Geometry: final body of the model. Coordinates: model frame, mm. A direction names the side the tool comes from. Coordinates: 2 decimals unless noted, no trailing zeros. Order: outer loops, then holes, each group sorted by start corner. A loop starts at its lowest first (then second) coordinate and runs counter-clockwise, first axis right, second up. Notation, with made-up numbers: M 14,28 L 19,28 A22 ccw 19,60 Z; hole C 13,25.5 d10. An arc over 180 degrees is marked long. Write item = value, one per line.
from build123d import *

# Parameters (mm, degrees)
ESQUISSE1_W             = 360
ESQUISSE1_H             = 356
BOSS_EXTRU_1_DEPTH      = 47.5
CONG_1_R                = 25
ENL_V_MAT_EXTRU_1_DEPTH = 44.5
ESQUISSE3_W             = 320
ESQUISSE3_H             = 35
ENL_V_MAT_EXTRU_2_DEPTH = 10
ESQUISSE5_W             = 40
ESQUISSE5_H             = 40
ESQUISSE5_W_2           = 34
ESQUISSE5_H_2           = 34
EXTRU_MINCE1_DEPTH      = 9.5
ESQUISSE10_W            = 34
ESQUISSE10_H            = 9.5
ENL_V_MAT_EXTRU_4_DEPTH = 10
ESQUISSE13_W            = 34
ESQUISSE13_H            = 9.5
ENL_V_MAT_EXTRU_5_DEPTH = 10


with BuildPart() as part:
    # Esquisse1 → Boss.-Extru.1 (new body)
    with BuildSketch(Plane.XY):
        with Locations((180, 178)):
            Rectangle(ESQUISSE1_W, ESQUISSE1_H)
    extrude(amount=BOSS_EXTRU_1_DEPTH)

    # Congé1
    cong_1_edges = [part.edges().sort_by_distance(p)[0] for p in [
        (0, 356, 23.75),
        (360, 356, 23.75),
        (360, 0, 23.75),
        (0, 0, 23.75),
    ]]
    fillet(cong_1_edges, radius=CONG_1_R)

    # Esquisse2 → Enlèv. mat.-Extru.1 (cut)
    with BuildSketch(Plane.XY.offset(47.5)):
        with BuildLine():
            Line((3, 331), (3, 25))
            ThreePointArc((3, 25), (9.443650814, 9.443650814), (25, 3))
            Line((25, 3), (335, 3))
            ThreePointArc((335, 3), (350.556349186, 9.443650814), (357, 25))
            Line((357, 25), (357, 331))
            ThreePointArc((357, 331), (350.556349186, 346.556349186), (335, 353))
            Line((335, 353), (25, 353))
            ThreePointArc((25, 353), (9.443650814, 346.556349186), (3, 331))
        make_face()
    extrude(amount=-ENL_V_MAT_EXTRU_1_DEPTH, mode=Mode.SUBTRACT)

    # Esquisse3 → Enlèv. mat.-Extru.2 (cut)
    with BuildSketch(Plane(origin=(0, 356, 0), x_dir=(1, 0, 0), z_dir=(0, 1, 0))):
        with Locations((180, -30)):
            Rectangle(ESQUISSE3_W, ESQUISSE3_H)
    extrude(amount=-ENL_V_MAT_EXTRU_2_DEPTH, mode=Mode.SUBTRACT)

    # Esquisse5 → Extru.-Mince1 (add)
    with BuildSketch(Plane.XY.offset(3)):
        with Locations((63, 333)):
            Rectangle(ESQUISSE5_W, ESQUISSE5_H)
        with Locations((63, 333)):
            Rectangle(ESQUISSE5_W_2, ESQUISSE5_H_2, mode=Mode.SUBTRACT)
        with Locations((297, 333)):
            Rectangle(ESQUISSE5_W, ESQUISSE5_H)
        with Locations((297, 333)):
            Rectangle(ESQUISSE5_W_2, ESQUISSE5_H_2, mode=Mode.SUBTRACT)
    extrude(amount=EXTRU_MINCE1_DEPTH)

    # Esquisse10 → Enlèv. mat.-Extru.4 (cut)
    with BuildSketch(Plane(origin=(0, 356, 0), x_dir=(1, 0, 0), z_dir=(0, 1, 0))):
        with Locations((297, -7.75)):
            Rectangle(ESQUISSE10_W, ESQUISSE10_H)
    extrude(amount=-ENL_V_MAT_EXTRU_4_DEPTH, mode=Mode.SUBTRACT)

    # Esquisse13 → Enlèv. mat.-Extru.5 (cut)
    with BuildSketch(Plane(origin=(0, 356, 0), x_dir=(1, 0, 0), z_dir=(0, 1, 0))):
        with Locations((63, -7.75)):
            Rectangle(ESQUISSE13_W, ESQUISSE13_H)
    extrude(amount=-ENL_V_MAT_EXTRU_5_DEPTH, mode=Mode.SUBTRACT)


solid = part.part
1) Section A-A, the plane y = 54. Return loops of the section in (x, z), and give its area (3 significant figures).
Numbers:
outline = M 0,0 L 360,0 L 360,47.5 L 357,47.5 L 357,3 L 3,3 L 3,47.5 L 0,47.5 Z
area = 1,350 mm²
2) Set-up query: faces 4 (the face through (352.482, 7.129, 24.082)), 5 (the face through (3, 180, 26)), 6 (the face through (63, 316, 8)). Return all of +Z, -Z, +X, -X, +Y, -Y with unobstructed straight access to the full face (end or side cutting, diameter ignored); none if empty.
Numbers:
face_4 = +Z, -Z, +X, -Y
face_5 = +Z
face_6 = +Z, +Y
3) Mould query, pull axis X, two halves, no side actions, for faces 1 (the face through (0, 176, 23)), 2 (the face through (178, 0, 23)), 3 (the face through (357, 176, 26)). Classes: pulls with the +X half, pulls with the -X half, needs draft (parallel to the pull), parting line crosses it, or undercut.
Numbers:
face_1 = pulls with the -X half
face_2 = needs draft
face_3 = undercut
4) Line query: L1, parallel to X at y = 132, z = 33; L2, parallel to Y at x = 65, z = 9.5; L3, parallel to Y at x = 186, z = 7. Output: solid intervals per line, ascending.
Numbers:
L1 = 0 to 3, 357 to 360
L2 = 0 to 3, 313 to 316
L3 = 0 to 3, 353 to 356
5) Section B-B, the plane x = 166. Return loops of the section in (y, z).
Numbers:
outline = M 0,0 L 356,0 L 356,12.5 L 353,12.5 L 353,3 L 3,3 L 3,47.5 L 0,47.5 Z
6) Pin query (flat end, axial travel): pin 1 (5 mm diameter, centred on y = 343, z = 6.5, fed in from +X); pin 2 (7.5 mm diameter, centred on x = 59.5, z = 7.5, fed in from +Y); pin 3 (5 mm diameter, centred on y = 336.5, z = 6.5, fed in from -X). Return the tip coordinate at first contact, or that it passes through.
Numbers:
pin_1 = 358.12
pin_2 = 316
pin_3 = 0.18
7) Section C-C, the plane z = 30. Return loops of the section in (x, y).
Numbers:
outline = M 0,25 A25 ccw 25,0 L 335,0 A25 ccw 360,25 L 360,331 A25 ccw 340,355.49 L 340,352.42 A22 cw 357,331 L 357,25 A22 cw 335,3 L 25,3 A22 cw 3,25 L 3,331 A22 cw 20,352.42 L 20,355.49 A25 ccw 0,331 Z
